```python
from build123d import *

# Parameters (mm, degrees)
F0_R     = 4
F1_DEPTH = 3
F2_R     = 12.5
F3_R     = 12.5


with BuildPart() as f1:
    # F0 (on Right) → F1 (new body)
    with BuildSketch(Plane.YZ):
        with BuildLine():
            Line((-241.300457, 281.4474), (-135.23444, 175.381383))
            Line((-135.23444, 175.381383), (-110.23444, 175.381383))
            Line((-110.23444, 175.381383), (-110.23444, 185.736722))
            Line((-110.23444, 185.736722), (-216.300457, 291.802739))
            Line((-216.300457, 291.802739), (-216.300457, 722.881383))
            ThreePointArc((-216.300457, 722.881383), (-219.961622, 731.720217), (-228.800457, 735.381383))
            ThreePointArc((-228.800457, 735.381383), (-237.639292, 731.720217), (-241.300457, 722.881383))
            Line((-241.300457, 722.881383), (-241.300457, 281.4474))
        make_face()
        with Locations((-228.800457, 722.881383)):
            Circle(F0_R, mode=Mode.SUBTRACT)
        with BuildLine():
            Line((-110.23444, 175.381383), (-135.23444, 175.381383))
            Line((-135.23444, 175.381383), (-135.23444, -127.118617))
            ThreePointArc((-135.23444, -127.118617), (-131.573275, -135.957452), (-122.73444, -139.618617))
            ThreePointArc((-122.73444, -139.618617), (-113.895605, -135.957452), (-110.23444, -127.118617))
            Line((-110.23444, -127.118617), (-110.23444, 175.381383))
        make_face()
        with Locations((-122.73444, -127.118617)):
            Circle(F0_R, mode=Mode.SUBTRACT)
        with Locations((-122.73444, 162.881383)):
            Circle(F0_R, mode=Mode.SUBTRACT)
    extrude(amount=F1_DEPTH)

    # F2
    f2_edges = [f1.edges().sort_by_distance(p)[0] for p in [
        (1.5, -110.23444, 185.736722),
        (1.5, -241.300457, 281.4474),
    ]]
    fillet(f2_edges, radius=F2_R)

    # F3
    f3_edges = [f1.edges().sort_by_distance(p)[0] for p in [
        (1.5, -135.23444, 175.381383),
        (1.5, -216.300457, 291.802739),
    ]]
    fillet(f3_edges, radius=F3_R)


solid = f1.part
```
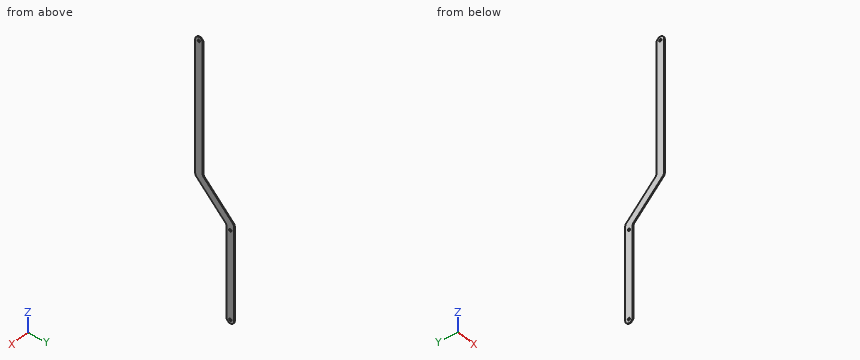
Source: CAD feature listing. Evaluate the final solid. Frame: model axes, mm. Coordinates: 2 decimals unless noted, no trailing zeros. Loops run counter-clockwise (first coordinate to the right, second up) from the corner with the lowest first, then second, coordinate; pieces in that order, holes last. Notation, with made-up numbers: M 4,22 L 48,22 A17 cw 48,55 Z; hole C -38,14.5 d3. An arc over 180 degrees is marked long. Put each result on its own line as item: value. Start each with the question number.
1) Ray query, L1, parallel to Y at x = 0.55, z = -9.5; L2, parallel to Y at x = 2, z = 408; L3, parallel to Y at x = 0.6, z = 159.5. Return the intervals inside material, ascending. Write a range as from..to.
2) Cut plane C-C on y = -200. Return the cut outline in (x, z).
3) Contact query for flat-ended pins moving along their axis: pin 1 Ø1.5 at (x, z) = (1, 85.5) entering from -Y; pin 2 Ø13 at (y, z) = (-122.73, 162.88) entering from +X. Output: stop coordinate, or through.
4) Cut plane A-A on x = 1.1. Return the cut outline in (y, z).
5) Cut plane B-B on z = 339. Return the cut outline in (x, y), then the cut area to 3 significant figures.
The answers:
1. L1: y = -135.23..-110.23
1. L2: y = -241.3..-216.3
1. L3: y = -135.23..-124.87, -120.6..-110.23
2. outline: M 0,240.15 L 3,240.15 L 3,275.5 L 0,275.5 Z
3. pin 1: stops at y = -135.23
3. pin 2: stops at x = 3
4. outline: M -241.3,286.63 A12.5 ccw -237.64,277.79 L -138.9,179.04 A12.5 cw -135.23,170.2 L -135.23,-127.12 A12.5 ccw -122.73,-139.62 A12.5 ccw -110.23,-127.12 L -110.23,180.56 A12.5 ccw -113.9,189.4 L -212.64,288.14 A12.5 cw -216.3,296.98 L -216.3,722.88 A12.5 ccw -228.8,735.38 A12.5 ccw -241.3,722.88 Z; hole C -228.8,722.88 d8; hole C -122.73,-127.12 d8; hole C -122.73,162.88 d8
5. outline: M 0,-241.3 L 3,-241.3 L 3,-216.3 L 0,-216.3 Z
5. area: 75.0 mm²
